```python
from build123d import *

# Parameters (mm, degrees)
F0_W     = 150
F0_H     = 100
F1_DEPTH = 15
F2_R     = 5
F3_T     = -2
F4_R     = 11.751583661
F5_DEPTH = 25


# Not quite as in the source:
# - a shell that OpenCascade refuses in one call is made with other operations: the cavity is built on its own and cut out


with BuildPart() as f1:
    # F0 (on Top) → F1 (new body)
    with BuildSketch(Plane.XY):
        Rectangle(F0_W, F0_H)
    extrude(amount=F1_DEPTH)

    # F2
    f2_edges = [f1.edges().sort_by_distance(p)[0] for p in [
        (0, 50, 0),
        (75, 0, 15),
        (0, 50, 15),
        (-75, 0, 15),
        (0, -50, 15),
        (-75, 50, 7.5),
        (-75, -50, 7.5),
        (-75, 0, 0),
        (75, -50, 7.5),
        (0, -50, 0),
        (75, 50, 7.5),
        (75, 0, 0),
    ]]
    fillet(f2_edges, radius=F2_R)

    # F3: a shell. OpenCascade refuses it in one call, so the cavity is built on its own and cut out:
    # the body offset inwards by the wall thickness, plus a prism from it out through each open face.
    f3_core = offset(f1.part, amount=F3_T, mode=Mode.PRIVATE)
    f3_exits = [f3_core.faces().sort_by_distance(p)[0] for p in [
        (0, 0, 2),
    ]]
    add(f3_core, mode=Mode.SUBTRACT)
    extrude(f3_exits, amount=-F3_T, mode=Mode.SUBTRACT)

    # F4 (on face) → F5 (cut)
    with BuildSketch(Plane.XY.offset(15)):
        with Locations((-47.0996387303, 0)):
            Circle(F4_R)
    extrude(amount=-F5_DEPTH, mode=Mode.SUBTRACT)


solid = f1.part
```
Verification items for the finished model (mm, model axes). A direction names the side the tool comes from. Coordinates: 2 decimals unless noted, no trailing zeros. Order: outer loops, then holes, each group sorted by start corner. A loop starts at its lowest first (then second) coordinate and runs counter-clockwise, first axis right, second up. Notation, with made-up numbers: (-2, -6) -> (20, -6) arc R27 cw to (20, 15) -> close; hole circle Ø1 at (17, 86). An arc over 180 degrees is marked (long way). Answer as CSV lines item,"result". Start each with the question number.
1) Gauge pin test, flat ends, axial feed: pin 1 Ø2 at (y, z) = (-15, 0.5) entering from +X; pin 2 Ø2 at (x, y) = (-7, -2.5) entering from -Z; pin 3 Ø1.6 at (x, z) = (-22.5, 1.5) entering from +Y. Record the tip position at first contact, or that the pin passes through.
2) Cross-section at B-B, the plane y = -40. Record the boundary of the cut face in (x, z).
3) Release check for a two-part mould opening along Y. For faces 1 (the face through (72.14, 0.63, 12.1)), 2 (the face through (1, 49, 2)), 3 (the face through (-74, 1, 13)), 4 (the face through (0.98, -47.14, 2.9)) record: released by +Y, released by -Y, zero draft, split by the parting line, or undercut.
4) Material ranges on L1, parallel to Y at x = 61.5, z = 9.5; L2, parallel to X at y = -42.5, z = 6; L3, parallel to Z at x = 29.5, y = -1, recorded low to high. Write a range as [from, to].
5) Cross-section at C-C, the plane x = 30.5. Record the boundary of the cut face in (y, z), then the cut area to 3 significant figures.
6) Set-up check for faces 5 (the face through (-74, -48, 8)), 6 (the face through (-72.14, 47.1, 7.54)): record each of +Z, -Z, +X, -X, +Y, -Y from which the full face is reachable in a straight line by a thin tool's end or side.
7) Cross-section at A-A, the plane y = 0. Record the boundary of the cut face in (x, z), then the cut area to 3 significant figures.
Conclusion:
1,pin 1,"stops at x = 73.57"
1,pin 2,"stops at z = 13"
1,pin 3,"stops at y = 49.21"
2,outline,"(-75, 5) arc R5 ccw to (-70, 0) -> (-70, 2) arc R3 cw to (-73, 5) -> (-73, 10) arc R3 cw to (-70, 13) -> (70, 13) arc R3 cw to (73, 10) -> (73, 5) arc R3 cw to (70, 2) -> (70, 0) arc R5 ccw to (75, 5) -> (75, 10) arc R5 ccw to (70, 15) -> (-70, 15) arc R5 ccw to (-75, 10) -> close"
3,face 1,"undercut"
3,face 2,"released by +Y"
3,face 3,"zero draft"
3,face 4,"undercut"
4,L1,"y = [-50, -48], [48, 50]"
4,L2,"x = [-75, -73], [73, 75]"
4,L3,"z = [13, 15]"
5,outline,"(-50, 5) arc R5 ccw to (-45, 0) -> (-45, 2) arc R3 cw to (-48, 5) -> (-48, 10) arc R3 cw to (-45, 13) -> (45, 13) arc R3 cw to (48, 10) -> (48, 5) arc R3 cw to (45, 2) -> (45, 0) arc R5 ccw to (50, 5) -> (50, 10) arc R5 ccw to (45, 15) -> (-45, 15) arc R5 ccw to (-50, 10) -> close"
5,area,"250 mm²"
6,face 5,"+Z, -Z, -X, -Y"
6,face 6,"none"
7,outline,"(-75, 5) arc R5 ccw to (-70, 0) -> (-70, 2) arc R3 cw to (-73, 5) -> (-73, 10) arc R3 cw to (-70, 13) -> (-58.85, 13) -> (-58.85, 15) -> (-70, 15) arc R5 ccw to (-75, 10) -> close; (-35.35, 13) -> (70, 13) arc R3 cw to (73, 10) -> (73, 5) arc R3 cw to (70, 2) -> (70, 0) arc R5 ccw to (75, 5) -> (75, 10) arc R5 ccw to (70, 15) -> (-35.35, 15) -> close"
7,area,"303 mm²"
